Could you check a few things on this drawing? It's one solid part, dimensions in mm from its lowest x, y, z. A direction names the side the tool comes from. Give positions to 0.01 mm unless a question says otherwise; leave off trailing zeros. Write item = value, one per line.
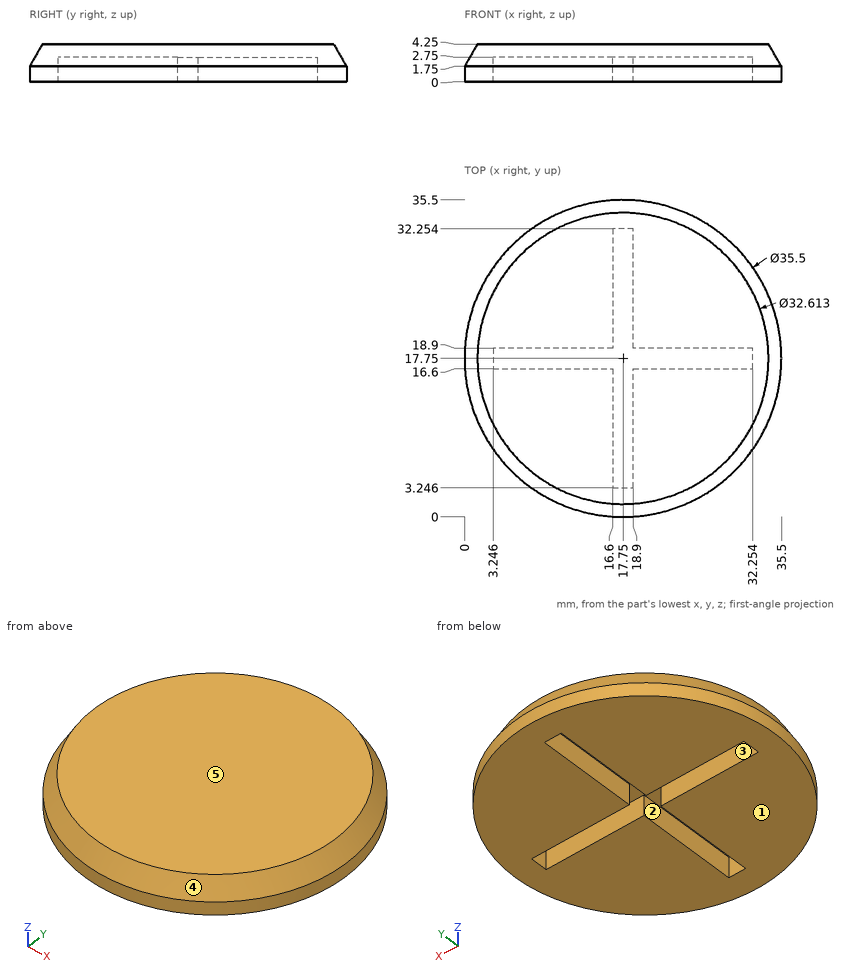
Q1. For pin 1 (2 mm diameter, centred on y = 9.5, z = 1.5, fed in from +X); pin 2 (1.4 mm diameter, centred on x = 12.5, z = 1.5, fed in from +Y); pin 3 (1 mm diameter, centred on x = 5.5, z = 3, fed in from +Y); pin 4 (1.5 mm diameter, centred on x = 4.5, y = 28, fed in from +Z), each with a flat end and sliding along its axis, tell me the tip position at first contact or that it passes through.
Output:
pin_1 = 33.95
pin_2 = 34.91
pin_3 = 30.22
pin_4 = 4.25
Q2. I need wall thicknesses on L1, parallel to Z at x = 17, y = 11; L2, parallel to X at y = 14.5, z = 0.4; L3, parallel to Y at x = 29, z = 0.4. Which ranges of each line are inside material? Lowest first, please.
Output:
L1 = 2.75 to 4.25
L2 = 0.3 to 16.6, 18.9 to 35.2
L3 = 4.02 to 16.6, 18.9 to 31.48
Q3. We'd pull the mould along Y, two halves only. Please class the marked faces 3, 4 and 5: released by +Y, released by -Y, zero draft, split by the parting line, or undercut.
Output:
face_3 = undercut
face_4 = split by the parting line
face_5 = zero draft
Q4. Which directions (+Z, -Z, +X, -X, +Y, -Y) give clear straight access to the entire face, cutting with the end or side of a thin tool? Please do the marked faces 1 and 2.
Output:
face_1 = -Z, +X, -X, +Y, -Y
face_2 = -Z
